from build123d import *

# Parameters (mm, degrees)
BOSS_EXTRU_1_DEPTH = 25


with BuildPart() as part:
    # Esquisse1 → Boss.-Extru.1 (new body)
    with BuildSketch(Plane.XY):
        with BuildLine():
            Line((20.572515541, 7.900512418), (17.017773047, 7.900512418))
            ThreePointArc((17.017773047, 7.900512418), (16.320544854, 8.183663168), (16.018158033, 8.872766723))
            Line((16.018158033, 8.872766723), (15.544759308, 25.928258114))
            ThreePointArc((15.544759308, 25.928258114), (14.545516715, 26.900512349), (13.545550223, 25.929002661))
            Line((13.545550223, 25.929002661), (13.057346636, 8.800141519))
            ThreePointArc((13.057346636, 8.800141519), (10.626813081, 6.400811923), (8.122740807, 8.723288601))
            Line((8.122740807, 8.723288601), (7.093366706, 25.96257467))
            ThreePointArc((7.093366706, 25.96257467), (6.095144481, 26.90297005), (5.096922241, 25.962574687))
            Line((5.096922241, 25.962574687), (4.067547777, 8.723288571))
            ThreePointArc((4.067547777, 8.723288571), (1.563475481, 6.400811945), (-0.867058048, 8.80014154))
            Line((-0.867058048, 8.80014154), (-1.355261635, 25.929002682))
            ThreePointArc((-1.355261635, 25.929002682), (-2.355228127, 26.90051237), (-3.35447072, 25.928258135))
            Line((-3.35447072, 25.928258135), (-3.827869445, 8.872766744))
            ThreePointArc((-3.827869445, 8.872766744), (-4.130256266, 8.183663189), (-4.827484459, 7.90051244))
            Line((-4.827484459, 7.90051244), (-8.382226953, 7.90051244))
            ThreePointArc((-8.382226953, 7.90051244), (-9.079455146, 8.183663189), (-9.381841967, 8.872766744))
            Line((-9.381841967, 8.872766744), (-9.855240692, 25.928258135))
            ThreePointArc((-9.855240692, 25.928258135), (-10.854483285, 26.90051237), (-11.854449777, 25.929002682))
            Line((-11.854449777, 25.929002682), (-12.355667565, 8.343531954))
            ThreePointArc((-12.355667565, 8.343531954), (-14.354855706, 6.40051244), (-16.354043847, 8.343531954))
            Line((-16.354043847, 8.343531954), (-16.855261635, 25.929002682))
            ThreePointArc((-16.855261635, 25.929002682), (-17.85338443, 26.900511357), (-18.854361615, 25.931943913))
            Line((-18.854361615, 25.931943913), (-19.42196512, 7.882422286))
            ThreePointArc((-19.42196512, 7.882422286), (-20.936113293, 6.400586914), (-22.479206535, 7.852256299))
            Line((-22.479206535, 7.852256299), (-23.406164612, 25.951660244))
            ThreePointArc((-23.406164612, 25.951660244), (-24.430437981, 26.90018516), (-25.404855706, 25.90051244))
            Line((-25.404855706, 25.90051244), (-25.404855706, 1.90051244))
            Line((-25.404855706, 1.90051244), (37.595144294, 1.90051244))
            Line((37.595144294, 1.90051244), (37.595144294, 25.900512418))
            ThreePointArc((37.595144294, 25.900512418), (36.620726569, 26.900185138), (35.5964532, 25.951660223))
            Line((35.5964532, 25.951660223), (34.669495123, 7.852256277))
            ThreePointArc((34.669495123, 7.852256277), (33.126401881, 6.400586892), (31.612253708, 7.882422264))
            Line((31.612253708, 7.882422264), (31.044650203, 25.931943892))
            ThreePointArc((31.044650203, 25.931943892), (30.043673018, 26.900511336), (29.045550223, 25.929002661))
            Line((29.045550223, 25.929002661), (28.544332435, 8.343531933))
            ThreePointArc((28.544332435, 8.343531933), (26.545144294, 6.400512418), (24.545956153, 8.343531933))
            Line((24.545956153, 8.343531933), (24.044738365, 25.929002661))
            ThreePointArc((24.044738365, 25.929002661), (23.044771873, 26.900512349), (22.04552928, 25.928258114))
            Line((22.04552928, 25.928258114), (21.572130555, 8.872766723))
            ThreePointArc((21.572130555, 8.872766723), (21.269743734, 8.183663168), (20.572515541, 7.900512418))
        make_face()
    extrude(amount=BOSS_EXTRU_1_DEPTH)


solid = part.part
The model under review builds one solid part; all positions refer to its coordinate system, in mm. Round coordinates to 2 decimals unless told otherwise and drop trailing zeros. Loops run counter-clockwise (first coordinate to the right, second up) from the corner with the lowest first, then second, coordinate; pieces in that order, holes last. Notation, with made-up numbers: (-28, -26.5) -> (26, -26.5) arc R22 ccw to (26, -8.5) -> close; hole circle Ø11 at (55.25, 50). An arc over 180 degrees is marked (long way). One line per question, with ' | ' between items. Start each with the question number.
Item 1: Wall thickness on line 1 along Y through (x, z) = (26.5, 7.75); line 2 along Y through (x, z) = (23, 16.5): over which ranges is each line inside the solid? List them lowest first. Write a range as [from, to].
Item 2: Add section D-D, the plane x = 2.5. Write out the cut boundary in (y, z), then the cut area to 3 significant figures.
Item 3: Add section B-B, the plane x = 27.5. Write out the cut boundary in (y, z).
Item 4: Draft analysis for pull direction X (two halves, no side actions). For faces 1 (the face through (-25.405, 14, 12)), 2 (the face through (6, 1.901, 12)), 3 (the face through (1.6, 6.4, 12.3)), state which applies: +X half, -X half, draft (parallel to the pull), parting line (faces both ways), or undercut.
Item 5: For pin 1 (4 mm diameter, centred on x = 18.5, z = 9, fed in from +Y) (3 decimals); pin 2 (10 mm diameter, centred on x = 27, y = 24, fed in from +Z); pin 3 (1.1 mm diameter, centred on x = -6, z = 16, fed in from +Y); pin 4 (1.5 mm diameter, centred on x = 29.5, z = 6.5, fed in from +Y), all flat-tipped, find the tip position at first contact; note any pin that passes through.
Item 6: Add section A-A, the plane y = 18. Count the separate pieces of the cut face and the enclosed holes in it, then the cut area to 3 significant figures.
Return value:
1) line 1: y = [1.9, 6.4] | line 2: y = [1.9, 26.9]
2) outline: (1.9, 0) -> (6.57, 0) -> (6.57, 25) -> (1.9, 25) -> close | area: 117 mm2
3) outline: (1.9, 0) -> (6.64, 0) -> (6.64, 25) -> (1.9, 25) -> close
4) face 1: -X half | face 2: draft | face 3: undercut
5) pin 1: stops at y = 8.045 | pin 2: stops at z = 25 | pin 3: stops at y = 7.9 | pin 4: stops at y = 26.9
6) separate pieces: 9 | enclosed holes: 0 | area: 562 mm2
